Work out the finished part from the listing and answer in its coordinate system (mm). A direction names the side the tool comes from. Coordinates: 2 decimals unless noted, no trailing zeros. Loops run counter-clockwise (first coordinate to the right, second up) from the corner with the lowest first, then second, coordinate; pieces in that order, holes last. Notation, with made-up numbers: (44.25, -23.75) -> (80.25, -23.75) arc R23 cw to (80.25, -1.75) -> close; hole circle Ø11 at (81, -18). An arc over 180 degrees is marked (long way). Use a Markdown table: item, result.
from build123d import *

# Parameters (mm, degrees)
SKETCH1_R           = 3.1
BOSS_EXTRUDE1_DEPTH = 3.75
CUT_EXTRUDE1_DEPTH  = 5


with BuildPart() as part:
    # Sketch1 → Boss-Extrude1 (new, symmetric)
    with BuildSketch(Plane(origin=(0, 0, 0), x_dir=(1, 0, 0), z_dir=(0, 1, 0))):
        Polygon((0, -11.547005384), (10, -5.773502692), (10, 5.773502692), (0, 11.547005384), (-10, 5.773502692), (-10, -5.773502692), align=None)
        with Locations(Location((0, 0, 0), (0, 0, 270))):
            Circle(SKETCH1_R, mode=Mode.SUBTRACT)
    extrude(amount=BOSS_EXTRUDE1_DEPTH, both=True)

    # Sketch2 → Cut-Extrude1 (cut)
    with BuildSketch(Plane(origin=(0, 3.75, 0), x_dir=(1, 0, 0), z_dir=(0, 1, 0))):
        Polygon((0, 5.860105232), (-5.075, 2.930052616), (-5.075, -2.930052616), (0, -5.860105232), (5.075, -2.930052616), (5.075, 2.930052616), align=None)
    extrude(amount=-CUT_EXTRUDE1_DEPTH, mode=Mode.SUBTRACT)


solid = part.part
Q1. Determine the mould class of faces 3 (the flat face through (-2.502, 1.285, -4.416)), 4 (the flat face through (5.07, 0.05, -8.62)), 5 (the flat face through (-2.4, -3.75, 2.4)) for opening direction X: pulls with the +X half, pulls with the -X half, needs draft (parallel to the pull), parting line crosses it, or undercut.
Solved:
| item | result |
|---|---|
| face 3 | undercut |
| face 4 | pulls with the +X half |
| face 5 | needs draft |
Q2. Section C-C on y = -2 is taken. Determine the outline of the cut face in (x, z), and give its area (3 significant figures).
Solved:
| item | result |
|---|---|
| outline | (-10, -5.77) -> (0, -11.55) -> (10, -5.77) -> (10, 5.77) -> (0, 11.55) -> (-10, 5.77) -> close; hole circle Ø6.2 at (0, 0) |
| area | 316 mm² |
Q3. Section D-D on z = 3.5 is taken. Determine the outline of the cut face in (x, y).
Solved:
| item | result |
|---|---|
| outline | (-10, -3.75) -> (10, -3.75) -> (10, 3.75) -> (4.09, 3.75) -> (4.09, -1.25) -> (-4.09, -1.25) -> (-4.09, 3.75) -> (-10, 3.75) -> close |
Q4. Section B-B on y = 1.75 is taken. Determine the outline of the cut face in (x, z) (1 decimal), and give its area (3 significant figures).
Solved:
| item | result |
|---|---|
| outline | (-10, -5.8) -> (0, -11.5) -> (10, -5.8) -> (10, 5.8) -> (0, 11.5) -> (-10, 5.8) -> close; hole (-5.1, -2.9) -> (0, -5.9) -> (5.1, -2.9) -> (5.1, 2.9) -> (0, 5.9) -> (-5.1, 2.9) -> close |
| area | 257 mm² |
Q5. Given pin 1 Ø1.5 at (x, y) = (6.5, 2) entering from +Z; pin 2 Ø1.5 at (x, y) = (7, 1) entering from -Z; pin 3 Ø4 at (y, z) = (-1.5, -9) entering from +X; pin 4 Ø5 at (x, z) = (0, 0) entering from +Y, each flat-ended and moving along its own axis, determine where each tip first touches the part or whether it passes through.
Solved:
| item | result |
|---|---|
| pin 1 | z = 8.23 |
| pin 2 | z = -7.94 |
| pin 3 | x = 7.88 |
| pin 4 | through |
Q6. Consider line 1 (X direction, y = -2.45, z = 0); line 2 (Z direction, x = -0.25, y = 3.5); line 3 (X direction, y = 2.75, z = 5.75). Determine where each line is inside the solid, lowest interval first. Write a range as [from, to].
Solved:
| item | result |
|---|---|
| line 1 | [-10, -3.1], [3.1, 10] |
| line 2 | [-11.4, -5.72], [5.72, 11.4] |
| line 3 | [-10, -0.19], [0.19, 10] |
Q7. Section A-A on z = 0 is taken. Determine the outline of the cut face in (x, y) (3 decimals).
Solved:
| item | result |
|---|---|
| outline | (-10, -3.75) -> (-3.1, -3.75) -> (-3.1, -1.25) -> (-5.075, -1.25) -> (-5.075, 3.75) -> (-10, 3.75) -> close; (3.1, -3.75) -> (10, -3.75) -> (10, 3.75) -> (5.075, 3.75) -> (5.075, -1.25) -> (3.1, -1.25) -> close |
Q8. For faces 1 (the flat face through (-2.573, 1.285, 4.375)), 2 (the flat face through (10, 0, 0)), determine the directions among +Z, -Z, +X, -X, +Y, -Y from which every point of the face is accessible in a straight line to the end or side of a thin tool.
Solved:
| item | result |
|---|---|
| face 1 | +Y |
| face 2 | +Z, -Z, +X, +Y, -Y |
